from build123d import *

# Parameters (mm, degrees)
SKETCH1_W           = 6
SKETCH1_H           = 6
SKETCH1_W_2         = 25.4
SKETCH1_H_2         = 41.91
BOSS_EXTRUDE1_DEPTH = 6
SKETCH2_W           = 12.7
SKETCH2_H           = 29.21
CUT_EXTRUDE1_DEPTH  = 29.719366724


with BuildPart() as part:
    # Sketch1 → Boss-Extrude1 (new body)
    with BuildSketch(Plane.XY):
        with Locations((-15.7, 14.43)):
            Rectangle(SKETCH1_W, SKETCH1_H)
        Rectangle(SKETCH1_W_2, SKETCH1_H_2)
        with Locations((-15.7, -14.43)):
            Rectangle(SKETCH1_W, SKETCH1_H)
        with Locations((15.7, -14.43)):
            Rectangle(SKETCH1_W, SKETCH1_H)
        with Locations((15.7, 14.43)):
            Rectangle(SKETCH1_W, SKETCH1_H)
    extrude(amount=BOSS_EXTRUDE1_DEPTH)

    # Sketch2 → Cut-Extrude1 (cut, through all)
    with BuildSketch(Plane.XY.offset(6)):
        Rectangle(SKETCH2_W, SKETCH2_H)
    extrude(amount=-CUT_EXTRUDE1_DEPTH, mode=Mode.SUBTRACT)


solid = part.part
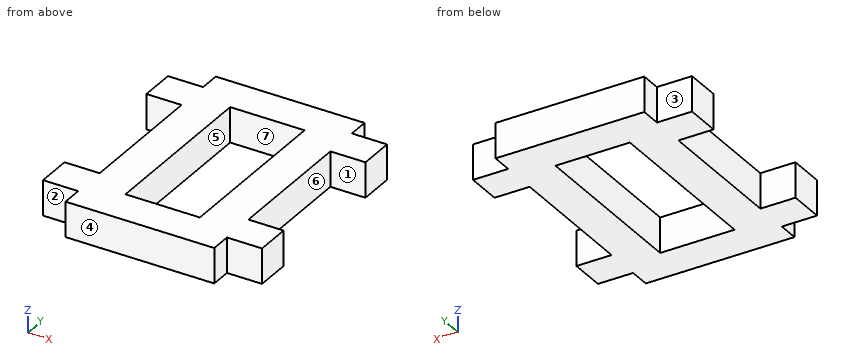
Could you check a few things on this model? Use its own coordinates, in mm. Face numbers are marked on the shaded views. A direction names the side the tool comes from. Round coordinates to 2 decimals unless told otherwise and drop trailing zeros. Order: outer loops, then holes, each group sorted by start corner. A loop starts at its lowest first (then second) coordinate and runs counter-clockwise, first axis right, second up.
(1) If we mould it in two halves opening along X, with no side actions, what happens to the marked faces 4, 5, 6 and 7? For each: released by +X, released by -X, zero draft, split by the parting line, or undercut.
Response values:
face 4: zero draft
face 5: undercut
face 6: released by +X
face 7: undercut
(2) Which directions (+Z, -Z, +X, -X, +Y, -Y) give clear straight access to the entire face, cutting with the end or side of a thin tool? Please do the marked faces 1, 2 and 3.
Response values:
face 1: +Z, -Z, +X
face 2: +Z, -Z, -X, -Y
face 3: +Z, -Z, -X, +Y
(3) I'm going to push flat-ended pins straight in: pin 1 (3 mm diameter, centred on y = -20, z = 3.5, fed in from -X); pin 2 (1 mm diameter, centred on y = -0.5, z = 5, fed in from +X); pin 3 (1.8 mm diameter, centred on x = -16, z = 3, fed in from +Y). Where does each tip first touch, or does it pass through?
Response values:
pin 1: stops at x = -12.7
pin 2: stops at x = 12.7
pin 3: stops at y = 17.43
(4) Please list where these lines run through material, in increasing order: line 1 along Y through (x, z) = (15, 2.7); line 2 along X through (y, z) = (-3.5, 4.8); line 3 along X through (y, z) = (12.5, 4.2).
Response values:
line 1: y = -17.43 to -11.43, 11.43 to 17.43
line 2: x = -12.7 to -6.35, 6.35 to 12.7
line 3: x = -18.7 to -6.35, 6.35 to 18.7
(5) Imagine slicing it at A-A (y = -8.5). Write out the boundary of the cut face in (x, z).
Response values:
outline: (-12.7, 0) - (-6.35, 0) - (-6.35, 6) - (-12.7, 6) - close; (6.35, 0) - (12.7, 0) - (12.7, 6) - (6.35, 6) - close
(6) Imagine slicing it at B-B (x = -3.5). Write out the boundary of the cut face in (y, z) (3 decimals).
Response values:
outline: (-20.955, 0) - (-14.605, 0) - (-14.605, 6) - (-20.955, 6) - close; (14.605, 0) - (20.955, 0) - (20.955, 6) - (14.605, 6) - close
(7) Imagine slicing it at C-C (z = 0.85). Write out the boundary of the cut face in (x, y) (3 decimals), plus the area to 3 significant figures.
Response values:
outline: (-18.7, -17.43) - (-12.7, -17.43) - (-12.7, -20.955) - (12.7, -20.955) - (12.7, -17.43) - (18.7, -17.43) - (18.7, -11.43) - (12.7, -11.43) - (12.7, 11.43) - (18.7, 11.43) - (18.7, 17.43) - (12.7, 17.43) - (12.7, 20.955) - (-12.7, 20.955) - (-12.7, 17.43) - (-18.7, 17.43) - (-18.7, 11.43) - (-12.7, 11.43) - (-12.7, -11.43) - (-18.7, -11.43) - close; hole (-6.35, -14.605) - (6.35, -14.605) - (6.35, 14.605) - (-6.35, 14.605) - close
area: 838 mm2
